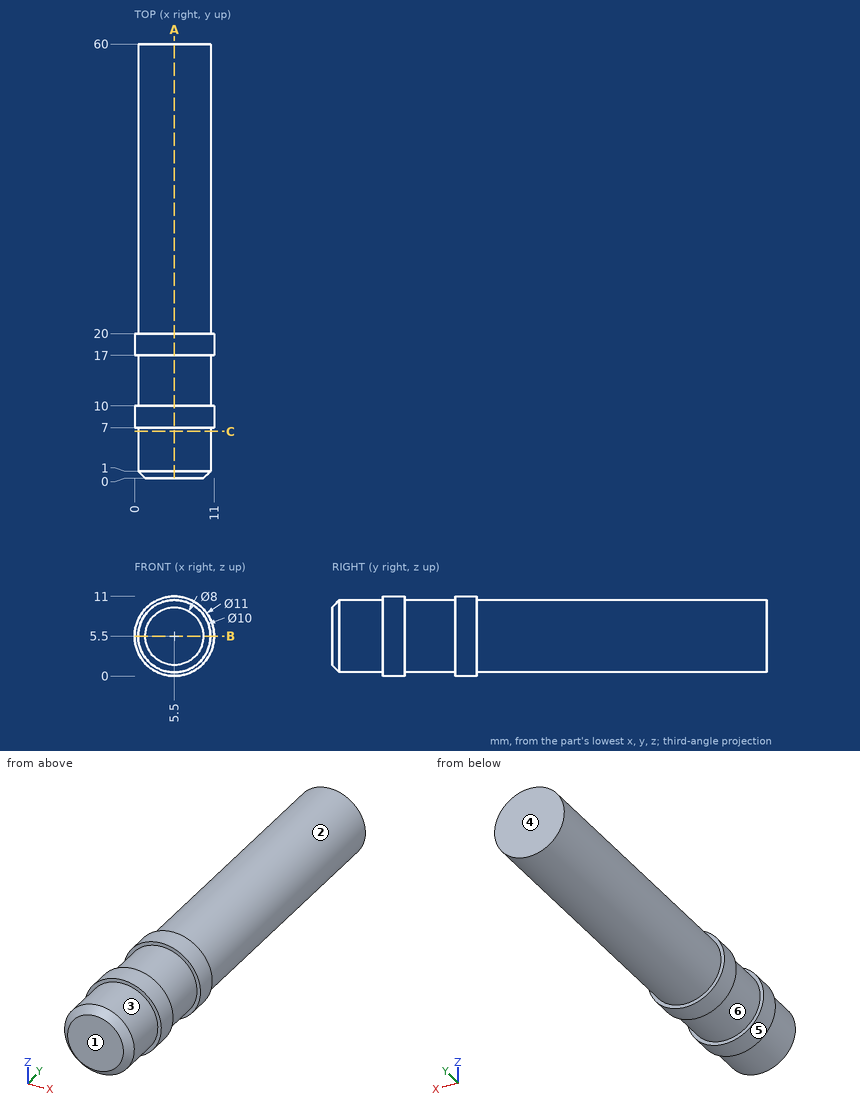
Job drawing, mm, ordinate dimensions from the low corner. One solid piece. A direction names the side the tool comes from. Coordinates: 2 decimals unless noted, no trailing zeros. Write each loop counter-clockwise with the first axis right and the second up, starting at its lowest first coordinate (ties: lowest second). Pieces come first, ordered by that corner, then holes. Notation, with made-up numbers: (-9.5, 43.25) -> (25.5, 43.25) arc R14 cw to (25.5, 49.25) -> close; hole circle Ø11 at (86, -24). An arc over 180 degrees is marked (long way). Use CSV: the item, a comma, the result in double quotes. Start each with the question number.
Item 1: Band-saw the part on A-A, the plane x = 5.5. Write the cut outline in (y, z), plus the area to 3 significant figures.
Item 2: Drop flat-ended pins along their axis: P1, Ø6, axis at x = 6.5, z = 5, coming from the -Y side; P2, Ø1, axis at y = 43.5, z = 5.5, coming from the +X side; P3, Ø4, axis at x = 9, y = 27, coming from the -Z side; P4, Ø2, axis at y = 13, z = 5.5, coming from the -X side. Give the stop position or say it passes through.
Item 3: Wall check: probe 1 along Y at (x, z) = (9, 1.75); probe 2 along Z at (x, y) = (8.5, 52). Give the ranges that are in metal, low to high.
Item 4: Tool access for the marked faces 1, 2 and 3: list every direction of +Z, -Z, +X, -X, +Y, -Y with a clear straight run to the whole face (end or side of a thin tool).
Item 5: Band-saw the part on C-C, the plane y = 6.5. Write the cut outline in (x, z).
Item 6: Band-saw the part on B-B, the plane z = 5.5. Write the cut outline in (x, y).
Item 7: Two-plate mould, pull along Y, no slides. Class the marked faces 4, 5 and 6: +Y half, -Y half, draft (parallel to the pull), parting line (faces both ways), or undercut.
Response values:
1,outline,"(0, 1.5) -> (1, 0.5) -> (7, 0.5) -> (7, 0) -> (10, 0) -> (10, 0.5) -> (17, 0.5) -> (17, 0) -> (20, 0) -> (20, 0.5) -> (60, 0.5) -> (60, 10.5) -> (20, 10.5) -> (20, 11) -> (17, 11) -> (17, 10.5) -> (10, 10.5) -> (10, 11) -> (7, 11) -> (7, 10.5) -> (1, 10.5) -> (0, 9.5) -> close"
1,area,"605 mm2"
2,P1,"stops at y = 0"
2,P2,"stops at x = 10.5"
2,P3,"stops at z = 0.73"
2,P4,"stops at x = 0.5"
3,probe 1,"y = 7 to 10, 17 to 20"
3,probe 2,"z = 1.5 to 9.5"
4,face 1,"+Z, -Z, +X, -X, -Y"
4,face 2,"+Y"
4,face 3,"-Y"
5,outline,"circle Ø10 at (5.5, 5.5)"
6,outline,"(0, 7) -> (0.5, 7) -> (0.5, 1) -> (1.5, 0) -> (9.5, 0) -> (10.5, 1) -> (10.5, 7) -> (11, 7) -> (11, 10) -> (10.5, 10) -> (10.5, 17) -> (11, 17) -> (11, 20) -> (10.5, 20) -> (10.5, 60) -> (0.5, 60) -> (0.5, 20) -> (0, 20) -> (0, 17) -> (0.5, 17) -> (0.5, 10) -> (0, 10) -> close"
7,face 4,"+Y half"
7,face 5,"draft"
7,face 6,"undercut"
